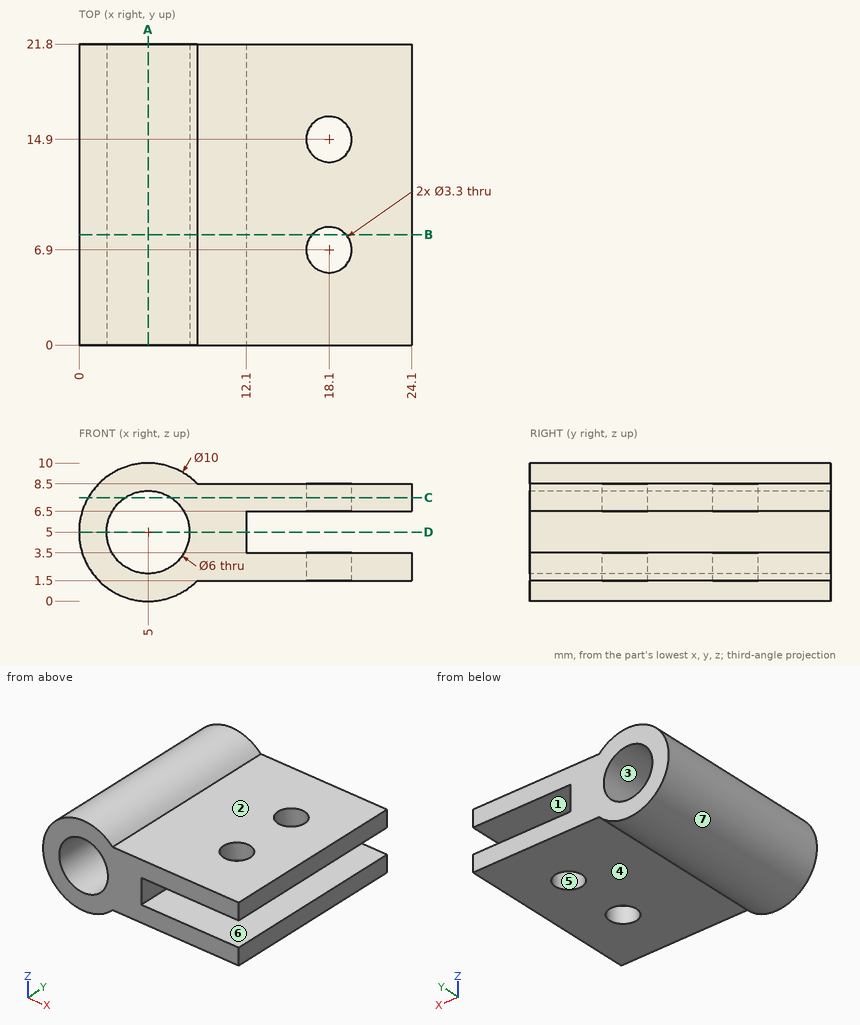
Answer from the drawing. Dimensions are ordinates in mm from the lowest x, y and z of the part. A direction names the side the tool comes from. Round coordinates to 2 decimals unless told otherwise and drop trailing zeros. Loops run counter-clockwise (first coordinate to the right, second up) from the corner with the lowest first, then second, coordinate; pieces in that order, holes last.
Q1. Determine the mould class of the marked faces 5, 6 and 7 for opening direction Z: released by +Z, released by -Z, zero draft, split by the parting line, or undercut.
Q2. Section C-C on z = 7.5 is taken. Write down the section's boundary in (x, y).
Q3. Section D-D on z = 5 is taken. Write down the section's boundary in (x, y), and give its area (3 significant figures).
Q4. Section A-A on x = 5 is taken. Write down the section's boundary in (y, z), and give its area (3 significant figures).
Q5. Section B-B on y = 8 is taken. Write down the section's boundary in (x, z).
Q6. Which of the six approach directions +Z, -Z, +X, -X, +Y, -Y give full straight-line access (tool end or side, diameter ignored) to the marked faces 1, 2, 3 and 4?
Q7. Each of these flat-tipped pins is pushed along its axis until it touches: pin 1 (10 mm diameter, centred on x = 16.5, y = 5, fed in from -Z); pin 2 (2 mm diameter, centred on x = 11, y = 14, fed in from +Z); pin 3 (5 mm diameter, centred on x = 5, z = 5, fed in from +Y); pin 4 (0.9 mm diameter, centred on y = 10, z = 5.5, fed in from +X). Where does it stop, or does it pass through?
Q8. Consider probe 1 along Y at (x, z) = (18.1, 2.7); probe 2 along Z at (x, y) = (18, 1.5); probe 3 along X at (y, z) = (3.25, 7.5). Determine where each line is inside the solid, lowest interval first.
Output:
1. face 5: zero draft
1. face 6: undercut
1. face 7: split by the parting line
2. outline: (0.67, 0) - (3.34, 0) - (3.34, 21.8) - (0.67, 21.8) - close; (6.66, 0) - (24.1, 0) - (24.1, 21.8) - (6.66, 21.8) - close; hole circle Ø3.3 at (18.1, 6.9); hole circle Ø3.3 at (18.1, 14.9)
3. outline: (0, 0) - (2, 0) - (2, 21.8) - (0, 21.8) - close; (8, 0) - (12.1, 0) - (12.1, 21.8) - (8, 21.8) - close
3. area: 133 mm2
4. outline: (0, 0) - (21.8, 0) - (21.8, 2) - (0, 2) - close; (0, 8) - (21.8, 8) - (21.8, 10) - (0, 10) - close
4. area: 87.2 mm2
5. outline: (8.57, 1.5) - (16.87, 1.5) - (16.87, 3.5) - (12.1, 3.5) - (12.1, 6.5) - (16.87, 6.5) - (16.87, 8.5) - (8.57, 8.5) arc R5 ccw (long way) to start; (19.33, 1.5) - (24.1, 1.5) - (24.1, 3.5) - (19.33, 3.5) - close; (19.33, 6.5) - (24.1, 6.5) - (24.1, 8.5) - (19.33, 8.5) - close; hole circle Ø6 at (5, 5)
6. face 1: +X, +Y, -Y
6. face 2: +Z, +X, +Y, -Y
6. face 3: +Y, -Y
6. face 4: -Z, +X, +Y, -Y
7. pin 1: stops at z = 1.5
7. pin 2: stops at z = 8.5
7. pin 3: passes through
7. pin 4: stops at x = 12.1
8. probe 1: y = 0 to 5.25, 8.55 to 13.25, 16.55 to 21.8
8. probe 2: z = 1.5 to 3.5, 6.5 to 8.5
8. probe 3: x = 0.67 to 3.34, 6.66 to 24.1
